Could you check a few things on this model? Use its own coordinates, in mm. A direction names the side the tool comes from. Coordinates: 2 decimals unless noted, no trailing zeros. Loops run counter-clockwise (first coordinate to the right, second up) from the corner with the lowest first, then second, coordinate; pieces in that order, holes last. Notation, with made-up numbers: (-19.5, -20) -> (-2.5, -20) arc R16 ccw to (-2.5, 7) -> close; hole circle Ø10 at (60, -34). An arc over 180 degrees is marked (long way). One line per question, with ' | ' between items.
```python
from build123d import *

# Parameters (mm, degrees)
CROSSRECESS_DEPTH = 2.6
FILLET5_R         = 0.3
HEADFILLET_R      = 1
DRAFT1_ANGLE      = 20


with BuildPart() as part:
    # Sketch1 → Base (revolve)
    with BuildSketch(Plane.XY):
        with BuildLine():
            Line((18.6, 2), (4, 2))
            Line((4, 2), (2.9, 2))
            ThreePointArc((2.9, 2), (2.687867966, 2.087867966), (2.6, 2.3))
            Line((2.6, 2.3), (2.6, 3.5))
            Line((2.6, 3.5), (0, 3.272529475))
            Line((0, 3.272529475), (0, 0))
            Line((0, 0), (18.6, 0))
            Line((18.6, 0), (18.6, 2))
        make_face()
    revolve(axis=Axis((4.515812911, 0, 0), (-1, 0, 0)))

    # Sketch6 → CrossRecess (cut)
    with BuildSketch(Plane(origin=(0, 0, 0), x_dir=(0, 0, -1), z_dir=(1, 0, 0))):
        Polygon((0.41, 0.41), (0.41, 2.05), (-0.41, 2.05), (-0.41, 0.41), (-2.05, 0.41), (-2.05, -0.41), (-0.41, -0.41), (-0.41, -2.05), (0.41, -2.05), (0.41, -0.41), (2.05, -0.41), (2.05, 0.41), align=None)
    extrude(amount=CROSSRECESS_DEPTH, mode=Mode.SUBTRACT)

    # Fillet5
    fillet5_edges = [part.edges().sort_by_distance(p)[0] for p in [
        (1.3, 0.41, 0.41),
        (1.3, -0.41, 0.41),
        (1.3, -0.41, -0.41),
        (1.3, 0.41, -0.41),
    ]]
    fillet(fillet5_edges, radius=FILLET5_R)

    # HeadFillet
    headfillet_edges = [part.edges().sort_by_distance(p)[0] for p in [
        (0, -3.272529475, 0),
    ]]
    fillet(headfillet_edges, radius=HEADFILLET_R)

    # Draft1
    draft1_faces = [part.faces().sort_by_distance(p)[0] for p in [
        (1.3, 0, 2.05),
        (1.3, -2.05, 0),
        (1.3, 0, -2.05),
        (1.3, 2.05, 0),
    ]]
    draft(draft1_faces, Plane(origin=(0, 0, 0), x_dir=(0, 0, -1), z_dir=(-1, 0, 0)), DRAFT1_ANGLE)


solid = part.part
```
Q1. Please list where these lines run through material, in increasing order: L1, parallel to Y at x = 15.25, z = 0; L2, parallel to X at y = 0.25, z = 0.5. Write a range as [from, to].
Values follow:
L1: y = [-2, 2] | L2: x = [2.6, 18.6]
Q2. For pin 1 (0.7 mm diameter, centred on x = 2, z = -1.5, fed in from -Y); pin 2 (1.5 mm diameter, centred on x = 1.5, y = 1.5, fed in from +Z); pin 3 (4 mm diameter, centred on y = 0.5, z = -0.5, fed in from -X); pin 4 (1.1 mm diameter, centred on x = 1.5, y = 1.5, fed in from -Z), each with a flat end and sliding along its axis, tell me the tip position at first contact or that it passes through.
Values follow:
pin 1: stops at y = -3.25 | pin 2: stops at z = 3.33 | pin 3: stops at x = 0 | pin 4: stops at z = -3.28
Q3. For faces 1 (the face through (11, 0, 2)), 2 (the face through (0, -1, -1)), 3 (the face through (1, -1, -0.41)), which set-ups out of +Z, -Z, +X, -X, +Y, -Y let a thin tool reach every point of the face, with its end or its side?
Values follow:
face 1: +X | face 2: +Z, -Z, -X, +Y, -Y | face 3: -X
Q4. Imagine slicing it at A-A on y = 0. Write out the boundary of the cut face in (x, z), plus the area to 3 significant figures.
Values follow:
outline: (0, -2.36) arc R1 ccw to (0.91, -3.35) -> (2.6, -3.5) -> (2.6, -2.3) arc R0.3 cw to (2.9, -2) -> (18.6, -2) -> (18.6, 2) -> (2.9, 2) arc R0.3 cw to (2.6, 2.3) -> (2.6, 3.5) -> (0.91, 3.35) arc R1 ccw to (0, 2.36) -> (0, 2.05) -> (2.6, 1.1) -> (2.6, -1.1) -> (0, -2.05) -> close | area: 73.1 mm2
Q5. We'd pull the mould along Y, two halves only. Please class faces 4 (the face through (1.37, -0.74, 3.31)), 5 (the face through (18.6, 0, 0)), 6 (the face through (1.282, -0.006, -1.583)), 7 (the face through (1, 1, 0.41)): released by +Y, released by -Y, zero draft, split by the parting line, or undercut.
Values follow:
face 4: split by the parting line | face 5: zero draft | face 6: undercut | face 7: undercut
Q6. Imagine slicing it at C-C on x = 13.75. Write out the boundary of the cut face in (y, z), plus the area to 3 significant figures.
Values follow:
outline: circle Ø4 at (0, 0) | area: 12.6 mm2
